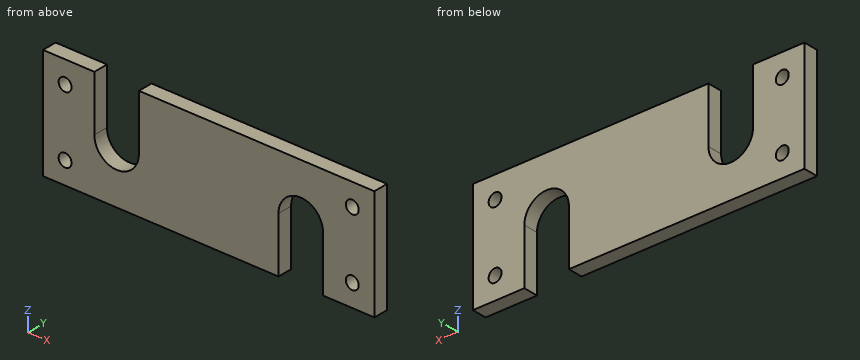
```python
from build123d import *

# Parameters (mm, degrees)
SKETCH2_W           = 90
SKETCH2_H           = 30
BOSS_EXTRUDE1_DEPTH = 4
SKETCH3_R           = 1.75
CUT_EXTRUDE1_DEPTH  = 5


with BuildPart() as part:
    # Sketch2 → Boss-Extrude1 (new body)
    with BuildSketch(Plane(origin=(0, 0, 0), x_dir=(1, 0, 0), z_dir=(0, 1, 0))):
        with Locations((45, 15)):
            Rectangle(SKETCH2_W, SKETCH2_H)
    extrude(amount=BOSS_EXTRUDE1_DEPTH)

    # Sketch3 → Cut-Extrude1 (cut, through all)
    with BuildSketch(Plane(origin=(0, 4, 0), x_dir=(1, 0, 0), z_dir=(0, 1, 0))):
        with Locations((6, 6)):
            Circle(SKETCH3_R)
        with Locations((6, 24)):
            Circle(SKETCH3_R)
        with Locations((84, 24)):
            Circle(SKETCH3_R)
        with Locations((84, 6)):
            Circle(SKETCH3_R)
        with BuildLine():
            Line((13.95, 0), (26.05, 0))
            Line((26.05, 0), (26.05, 15))
            ThreePointArc((26.05, 15), (20, 21.05), (13.95, 15))
            Line((13.95, 15), (13.95, 0))
        make_face()
        with BuildLine():
            Line((63.95, 30), (63.95, 15))
            ThreePointArc((63.95, 15), (70, 8.95), (76.05, 15))
            Line((76.05, 15), (76.05, 30))
            Line((76.05, 30), (63.95, 30))
        make_face()
    extrude(amount=-CUT_EXTRUDE1_DEPTH, mode=Mode.SUBTRACT)


solid = part.part
```
Geometry: final body of the model. Coordinates: model frame, mm. Give positions to 0.01 mm unless a question says otherwise; leave off trailing zeros. Write each loop counter-clockwise with the first axis right and the second up, starting at its lowest first coordinate (ties: lowest second). Pieces come first, ordered by that corner, then holes.
1. Line query: probe 1 along Z at (x, y) = (84, 1.85); probe 2 along X at (y, z) = (1.6, -6); probe 3 along X at (y, z) = (1.8, -24). Output: solid intervals per line, ascending.
2. Section query C-C, the plane x = 84. Return loops of the section in (y, z), then the cut area to 3 significant figures.
3. Section query B-B, the plane y = 2.8. Return loops of the section in (x, z), then the cut area to 3 significant figures.
4. Section query D-D, the plane z = -18.5. Return loops of the section in (x, y), then the cut area to 3 significant figures.
5. Section query A-A, the plane z = -27. Return loops of the section in (x, y).
Computed:
1. probe 1: z = -30 to -25.75, -22.25 to -7.75, -4.25 to 0
1. probe 2: x = 0 to 4.25, 7.75 to 13.95, 26.05 to 82.25, 85.75 to 90
1. probe 3: x = 0 to 4.25, 7.75 to 63.95, 76.05 to 82.25, 85.75 to 90
2. outline: (0, -30) - (4, -30) - (4, -25.75) - (0, -25.75) - close; (0, -22.25) - (4, -22.25) - (4, -7.75) - (0, -7.75) - close; (0, -4.25) - (4, -4.25) - (4, 0) - (0, 0) - close
2. area: 92.0 mm2
3. outline: (0, -30) - (63.95, -30) - (63.95, -15) arc R6.05 cw to (76.05, -15) - (76.05, -30) - (90, -30) - (90, 0) - (26.05, 0) - (26.05, -15) arc R6.05 cw to (13.95, -15) - (13.95, 0) - (0, 0) - close; hole circle Ø3.5 at (6, -24); hole circle Ø3.5 at (6, -6); hole circle Ø3.5 at (84, -24); hole circle Ø3.5 at (84, -6)
3. area: 2,180 mm2
4. outline: (0, 0) - (15.07, 0) - (15.07, 4) - (0, 4) - close; (24.93, 0) - (63.95, 0) - (63.95, 4) - (24.93, 4) - close; (76.05, 0) - (90, 0) - (90, 4) - (76.05, 4) - close
4. area: 272 mm2
5. outline: (0, 0) - (63.95, 0) - (63.95, 4) - (0, 4) - close; (76.05, 0) - (90, 0) - (90, 4) - (76.05, 4) - close
